```python
from build123d import *

# Parameters (mm, degrees)
SKETCH1_R                 = 19
SKETCH1_R_2               = 14
BOSS_EXTRUDE1_DEPTH       = 125
BOSS_EXTRUDE2_START       = 7.5
SKETCH2_R                 = 14
BOSS_EXTRUDE2_DEPTH       = 7.5
CUT_EXTRUDE1_DEPTH        = 121.53319045
CUT_EXTRUDE1_DEPTH_BACK   = 121.53319045
SKETCH4_R                 = 6.025
SKETCH5_R                 = 14
BOSS_EXTRUDE3_DEPTH       = 7.5
BOSS_EXTRUDE4_DEPTH       = 15
BOSS_EXTRUDE4_DEPTH_BACK  = 140
SKETCH7_R                 = 6.025
CUT_EXTRUDE2_DEPTH        = 143.555252446
CUT_EXTRUDE2_DEPTH_BACK   = 143.555252446
SKETCH8_R                 = 1.5
SKETCH9_R                 = 3.5
CUT_EXTRUDE3_DEPTH        = 22
SKETCH11_R                = 15
BOSS_EXTRUDE5_DEPTH       = 5
LPATTERN1_COUNT           = 2
LPATTERN1_PITCH           = 30
LPATTERN2_COPY_1_SKETCH_R = 15
LPATTERN2_COPY_1_DEPTH    = 5
LPATTERN2_COPY_2_SKETCH_R = 15
LPATTERN2_COPY_2_DEPTH    = 5


with BuildPart() as part:
    # Sketch1 → Boss-Extrude1 (new body)
    with BuildSketch(Plane.XY):
        Circle(SKETCH1_R)
        Circle(SKETCH1_R_2, mode=Mode.SUBTRACT)
    extrude(amount=-BOSS_EXTRUDE1_DEPTH)

    # Sketch2 → Boss-Extrude2 (add)
    with BuildSketch(Plane.XY.offset(-7.5).offset(BOSS_EXTRUDE2_START)):
        Circle(SKETCH2_R)
    extrude(amount=-BOSS_EXTRUDE2_DEPTH)

    # Sketch4 → Cut-Extrude1 (cut, two sides: drawn at the far end of the back side and taken through both)
    with BuildSketch(Plane.XY.offset(-7.5).offset(-CUT_EXTRUDE1_DEPTH_BACK)):
        Circle(SKETCH4_R)
    extrude(amount=CUT_EXTRUDE1_DEPTH + CUT_EXTRUDE1_DEPTH_BACK, mode=Mode.SUBTRACT)

    # Sketch5 → Boss-Extrude3 (add)
    with BuildSketch(Plane(origin=(0, 0, -117.5), x_dir=(-1, 0, 0), z_dir=(0, 0, -1))):
        with Locations(Location((0, 0, 0), (0, 0, 180))):
            Circle(SKETCH5_R)
    extrude(amount=BOSS_EXTRUDE3_DEPTH)

    # Sketch7 → Boss-Extrude4 (add, two sides: drawn at the far end of the back side and taken through both)
    with BuildSketch(Plane.XY.offset(-BOSS_EXTRUDE4_DEPTH_BACK)):
        Circle(SKETCH7_R)
    extrude(amount=BOSS_EXTRUDE4_DEPTH + BOSS_EXTRUDE4_DEPTH_BACK)

    # Sketch8 → Cut-Extrude2 (cut, two sides: drawn at the far end of the back side and taken through both)
    with BuildSketch(Plane(origin=(0, 0, 0), x_dir=(1, 0, 0), z_dir=(0, 1, 0)).offset(-CUT_EXTRUDE2_DEPTH_BACK)):
        with Locations(Location((0, 127.5, 0), (0, 0, 270))):
            Circle(SKETCH8_R)
    extrude(amount=CUT_EXTRUDE2_DEPTH + CUT_EXTRUDE2_DEPTH_BACK, mode=Mode.SUBTRACT)

    # Sketch9 → Cut-Extrude3 (cut)
    with BuildSketch(Plane(origin=(0, 0, -140), x_dir=(-1, 0, 0), z_dir=(0, 0, -1))):
        Circle(SKETCH9_R)
    extrude(amount=-CUT_EXTRUDE3_DEPTH, mode=Mode.SUBTRACT)

    # Sketch11 → Boss-Extrude5 (add, symmetric)
    with BuildSketch(Plane(origin=(0, 0, -62.5), x_dir=(-1, 0, 0), z_dir=(0, 0, -1))):
        Circle(SKETCH11_R)
    boss_extrude5 = extrude(amount=BOSS_EXTRUDE5_DEPTH, both=True)

    # LPattern1: Boss-Extrude5 ×2
    with Locations(*[(0, 0, -i * LPATTERN1_PITCH) for i in range(1, LPATTERN1_COUNT)]):
        add(boss_extrude5)

    # LPattern2 copy 1 sketch → LPattern2 copy 1 (add, symmetric)
    with BuildSketch(Plane(origin=(0, 0, -62.5), x_dir=(-1, 0, 0), z_dir=(0, 0, -1))):
        Circle(LPATTERN2_COPY_1_SKETCH_R)
    extrude(amount=LPATTERN2_COPY_1_DEPTH, both=True)

    # LPattern2 copy 2 sketch → LPattern2 copy 2 (add, symmetric)
    with BuildSketch(Plane(origin=(0, 0, -32.5), x_dir=(-1, 0, 0), z_dir=(0, 0, -1))):
        Circle(LPATTERN2_COPY_2_SKETCH_R)
    extrude(amount=LPATTERN2_COPY_2_DEPTH, both=True)


solid = part.part
```
Part model, mm, in its own coordinate system. A direction names the side the tool comes from. Round coordinates to 2 decimals unless told otherwise and drop trailing zeros. Order: outer loops, then holes, each group sorted by start corner. A loop starts at its lowest first (then second) coordinate and runs counter-clockwise, first axis right, second up. Notation, with made-up numbers: M -19.5,-27 L 30.5,-27 A19 cw 30.5,-6 Z; hole C 54.5,60 d10. An arc over 180 degrees is marked long. Answer in a Markdown table with one row per item. Add a question column.
Q1. Cut at D-D on z = -127.5. Give the cut face in (x, y) (3 decimals), and give its area (3 significant figures).
Q2. 3-axis set-ups, long thin cutter, end or side, ignore diameter. For faces 4 (the face through (5.747, 1.81, -132.605)), 5 (the face through (3, 6, -117.5)), 6 (the face through (0, 0, 15)): which of +Z, -Z, +X, -X, +Y, -Y reach the whole face in a straight line?
Q3. Wall check: L1, parallel to Z at x = -2.5, y = 6; L2, parallel to Y at x = 0, z = -12.75 (3 decimals); L3, parallel to X at y = -0.5, z = -102.5. Give the ranges that are in metal, low to high. Write a range as from..to.
Q4. Mould opens along X. For faces 1 (the face through (1.265, -4.616, -126.694)), 2 (the face through (3, -3, -140)), 3 (the face through (8.767, -16.856, -61.625)) say: +X half, -X half, draft (parallel to the pull), parting line (faces both ways), or undercut.
Q5. Cut at B-B on y = 10. Give the cut face in (x, z).
Q6. Pin check, flat tips, straight feed: pin 1 (8.5 mm diameter, centred on x = 6, y = 5, fed in from -Z); pin 2 (8 mm diameter, centred on x = 7, z = -86.5, fed in from +Y); pin 3 (12 mm diameter, centred on x = 13, y = 0.5, fed in from -Z); pin 4 (5 mm diameter, centred on y = 10, z = -107.5, fed in from -X). Stop position of each tip, or through.
Q7. Cut at C-C on x = 0. Give the number of separate pieces and of enclosed holes in the cut face, and give its area (3 significant figures).
Q8. Cut at A-A on z = -102.5. Give the cut face in (x, y) (3 decimals).
Established:
| question | item | result |
|---|---|---|
| 1 | outline | M -1.5,-5.835 L -1.5,-3.162 A3.5 cw -1.5,3.162 L -1.5,5.835 A6.025 ccw Z; M 1.5,-5.835 A6.025 ccw 1.5,5.835 L 1.5,3.162 A3.5 cw 1.5,-3.162 Z |
| 1 | area | 60.1 mm2 |
| 2 | face 4 | -Z |
| 2 | face 5 | none |
| 2 | face 6 | +Z, +X, -X, +Y, -Y |
| 3 | L1 | z = -125..-117.5, -97.5..-87.5, -67.5..-57.5, -37.5..-27.5, -7.5..0 |
| 3 | L2 | y = -19..-14, -6.025..6.025, 14..19 |
| 3 | L3 | x = -18.99..-13.99, -6..6, 13.99..18.99 |
| 4 | face 1 | undercut |
| 4 | face 2 | draft |
| 4 | face 3 | parting line |
| 5 | outline | M -16.16,-125 L 16.16,-125 L 16.16,0 L -16.16,0 Z; hole M -9.8,-117.5 L 9.8,-117.5 L 9.8,-97.5 L -9.8,-97.5 Z; hole M -9.8,-87.5 L 9.8,-87.5 L 9.8,-67.5 L -9.8,-67.5 Z; hole M -9.8,-57.5 L 9.8,-57.5 L 9.8,-37.5 L -9.8,-37.5 Z; hole M -9.8,-27.5 L 9.8,-27.5 L 9.8,-7.5 L -9.8,-7.5 Z |
| 6 | pin 1 | stops at z = -140 |
| 6 | pin 2 | stops at y = 18.76 |
| 6 | pin 3 | stops at z = -125 |
| 6 | pin 4 | stops at x = -17.46 |
| 7 | separate pieces | 3 |
| 7 | enclosed holes | 8 |
| 7 | area | 3,670 mm2 |
| 8 | outline | C 0,0 d38; C 0,0 d12.05; hole C 0,0 d28 |
